For this review, take the finished solid that the model builds, in its own axes (mm). Face numbers are marked on the shaded views. A direction names the side the tool comes from. Coordinates: 2 decimals unless noted, no trailing zeros. Loops run counter-clockwise (first coordinate to the right, second up) from the corner with the lowest first, then second, coordinate; pieces in that order, holes last. Notation, with made-up numbers: M 84.5,-18 L 130.5,-18 A12 ccw 130.5,-9 Z; hole C 13.25,50 d5. An arc over 180 degrees is marked long. Answer as a JSON object with one key per item and string values. Group by question number.
Item 1: Mouldability with a two-part tool opening along X and no side actions: class the marked faces 3, 4 and 5 as +X half, -X half, draft (parallel to the pull), parting line (faces both ways), or undercut.
Item 2: Wall thickness on L1, parallel to Y at x = 0, z = 6; L2, parallel to Y at x = 0, z = 0.4; L3, parallel to Y at x = 0, z = 0.2: over which ranges is each line inside the solid? List them lowest first. Write a range as from..to.
Item 3: Insertion check: pin 1 (12 mm diameter, centred on x = 0.5, y = -5.5, fed in from +Z); pin 2 (2 mm diameter, centred on x = -2.5, z = 8, fed in from -Y); pin 3 (5 mm diameter, centred on x = -10, z = 8.5, fed in from +Y); pin 4 (3 mm diameter, centred on x = 7, y = 8, fed in from +Z). Each pin has a flat end and moves straight along its axis. Give the tip position at first contact, or say it passes through.
Item 4: Add section C-C (z = 10.5). State the section outline as (x, y) points.
Item 5: Tool access review of the marked faces 1 and 2: name each direction out of +Z, -Z, +X, -X, +Y, -Y from which nothing blocks a thin tool from reaching the whole face with its end or side.
from build123d import *

# Parameters (mm, degrees)
F0_R     = 15
F0_R_2   = 5
F1_DEPTH = 14.3
F2_R     = 0.6
F3_R     = 13.85
F3_R_2   = 8.6
F4_DEPTH = 0.5
F5_R     = 13.85
F5_R_2   = 8.6
F6_DEPTH = 0.5


with BuildPart() as f1:
    # F0 (on Top) → F1 (new body)
    with BuildSketch(Plane.XY):
        Circle(F0_R)
        Circle(F0_R_2, mode=Mode.SUBTRACT)
    extrude(amount=F1_DEPTH)

    # F2
    f2_edges = [f1.edges().sort_by_distance(p)[0] for p in [
        (5, 0, 7.15),
        (-5, 0, 0),
        (-5, 0, 14.3),
        (15, 0, 7.15),
        (-15, 0, 0),
        (-15, 0, 14.3),
    ]]
    fillet(f2_edges, radius=F2_R)

    # F3 (on face) → F4 (cut)
    with BuildSketch(Plane.XY.offset(14.3)):
        Circle(F3_R)
        Circle(F3_R_2, mode=Mode.SUBTRACT)
    extrude(amount=-F4_DEPTH, mode=Mode.SUBTRACT)

    # F5 (on face) → F6 (cut)
    with BuildSketch(Plane(origin=(0, 0, 0), x_dir=(1, 0, 0), z_dir=(0, 0, -1))):
        Circle(F5_R)
        Circle(F5_R_2, mode=Mode.SUBTRACT)
    extrude(amount=-F6_DEPTH, mode=Mode.SUBTRACT)


solid = f1.part
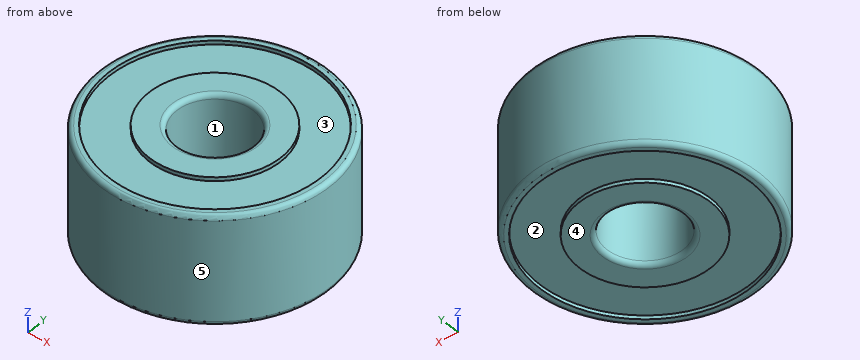
From the geometry:
{
 "1": {"face 3": "undercut", "face 4": "draft", "face 5": "parting line"},
 "2": {"L1": "y = -15..-5, 5..15", "L2": "y = -14.97..-13.85, -8.6..-5.03, 5.03..8.6, 13.85..14.97", "L3": "y = -14.85..-13.85, -8.6..-5.15, 5.15..8.6, 13.85..14.85"},
 "3": {"pin 1": "stops at z = 14.3", "pin 2": "stops at y = -14.92", "pin 3": "stops at y = 12.99", "pin 4": "stops at z = 13.8"},
 "4": {"outline": "C 0,0 d30; hole C 0,0 d10"},
 "5": {"face 1": "+Z, -Z", "face 2": "-Z"}
}
